from build123d import *

# Parameters (mm, degrees)
SKETCH1_W               = 25
SKETCH1_H               = 70
SKETCH1_R               = 7.6
SKETCH1_R_2             = 5.25
BOSS_EXTRUDE2_DEPTH     = 100
SKETCH1_12_R            = 1.575
CUT_EXTRUDE5_DEPTH      = 12.8
SKETCH1_27_R            = 11.15
CORTAR_EXTRUIR1_DEPTH   = 3.5
CROQUIS1_W              = 70
CROQUIS1_H              = 25
SALIENTE_EXTRUIR1_DEPTH = 150
CROQUIS4_R              = 29
CORTAR_EXTRUIR2_DEPTH   = 30
CUT_EXTRUDE6_START      = -25
CROQUIS4_3_W            = 12.3
CROQUIS4_3_H            = 22.718001441
CUT_EXTRUDE6_DEPTH      = 22
CUT_EXTRUDE7_START      = -25
CROQUIS4_4_R            = 1
CUT_EXTRUDE7_DEPTH      = 6
SKETCH2_W               = 12.2
SKETCH2_H               = 6.16
CUT_EXTRUDE11_DEPTH     = 28
CROQUIS5_R              = 2.6
CORTAR_EXTRUIR3_DEPTH   = 50


with BuildPart() as part:
    # Sketch1 → Boss-Extrude2 (new body)
    with BuildSketch(Plane(origin=(0, 0, 0), x_dir=(1, 0, 0), z_dir=(0, 1, 0))):
        Rectangle(SKETCH1_W, SKETCH1_H)
        with Locations((0, 21)):
            Circle(SKETCH1_R, mode=Mode.SUBTRACT)
        with Locations((0, -21)):
            Circle(SKETCH1_R, mode=Mode.SUBTRACT)
        Circle(SKETCH1_R_2, mode=Mode.SUBTRACT)
    extrude(amount=BOSS_EXTRUDE2_DEPTH)

    # Sketch1<12> → Cut-Extrude5 (cut)
    with BuildSketch(Plane(origin=(0, 0, 0), x_dir=(1, 0, 0), z_dir=(0, 1, 0))):
        with Locations((0, 8.193732966)):
            Circle(SKETCH1_12_R)
        with Locations((8.193732966, 0)):
            Circle(SKETCH1_12_R)
        with Locations((0, -8.193732966)):
            Circle(SKETCH1_12_R)
        with Locations((-8.193732966, 0)):
            Circle(SKETCH1_12_R)
    extrude(amount=CUT_EXTRUDE5_DEPTH, mode=Mode.SUBTRACT)

    # Sketch1<27> → Cortar-Extruir1 (cut)
    with BuildSketch(Plane(origin=(0, 0, 0), x_dir=(1, 0, 0), z_dir=(0, 1, 0))):
        Circle(SKETCH1_27_R)
    extrude(amount=CORTAR_EXTRUIR1_DEPTH, mode=Mode.SUBTRACT)

    # Croquis1 → Saliente-Extruir1 (add)
    with BuildSketch(Plane(origin=(12.5, 0, 0), x_dir=(0, 0, -1), z_dir=(1, 0, 0))):
        with Locations((0, 12.5)):
            Rectangle(CROQUIS1_W, CROQUIS1_H)
    extrude(amount=SALIENTE_EXTRUIR1_DEPTH)

    # Croquis4 → Cortar-Extruir2 (cut)
    with BuildSketch(Plane.XZ):
        with Locations((107.66, 0)):
            Circle(CROQUIS4_R)
    extrude(amount=-CORTAR_EXTRUIR2_DEPTH, mode=Mode.SUBTRACT)

    # Croquis4<3> → Cut-Extrude6 (cut)
    with BuildSketch(Plane.XZ.offset(CUT_EXTRUDE6_START)):
        with Locations((32.807294184, 12.912589049)):
            Rectangle(CROQUIS4_3_W, CROQUIS4_3_H)
    extrude(amount=CUT_EXTRUDE6_DEPTH, mode=Mode.SUBTRACT)

    # Croquis4<4> → Cut-Extrude7 (cut)
    with BuildSketch(Plane.XZ.offset(CUT_EXTRUDE7_START)):
        with Locations((32.807294184, -1.398410231)):
            Circle(CROQUIS4_4_R)
        with Locations((32.807294184, 26.301614952)):
            Circle(CROQUIS4_4_R)
    extrude(amount=CUT_EXTRUDE7_DEPTH, mode=Mode.SUBTRACT)

    # Sketch2 → Cut-Extrude11 (cut)
    with BuildSketch(Plane.XY.offset(35)):
        with Locations((32.75, 11.48)):
            Rectangle(SKETCH2_W, SKETCH2_H)
    extrude(amount=-CUT_EXTRUDE11_DEPTH, mode=Mode.SUBTRACT)

    # Croquis5 → Cortar-Extruir3 (cut)
    with BuildSketch(Plane(origin=(0, 25, 0), x_dir=(1, 0, 0), z_dir=(0, 1, 0))):
        with Locations((56.60021437, -13.16922633)):
            Circle(CROQUIS5_R)
        with Locations((56.60021437, 11.27722458)):
            Circle(CROQUIS5_R)
    extrude(amount=-CORTAR_EXTRUIR3_DEPTH, mode=Mode.SUBTRACT)


solid = part.part
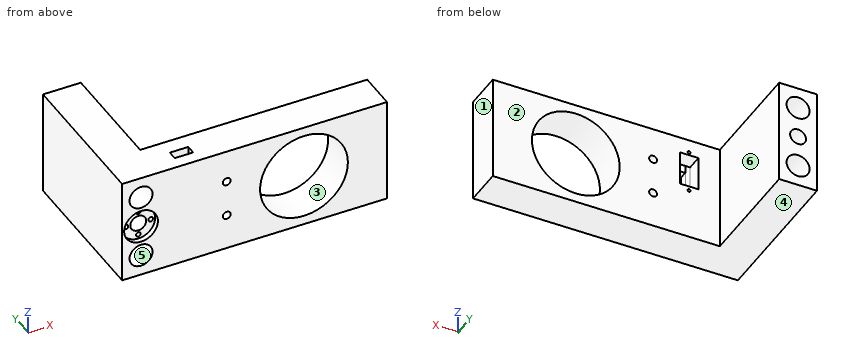
Work out the finished part from the listing and answer in its coordinate system (mm). Face numbers are marked on the shaded views. A direction names the side the tool comes from. Give positions to 0.01 mm unless a question says otherwise; leave off trailing zeros. Write each loop counter-clockwise with the first axis right and the second up, starting at its lowest first coordinate (ties: lowest second). Pieces come first, ordered by that corner, then holes. Notation, with made-up numbers: (68.5, 5) - (85.5, 5) arc R25 cw to (85.5, 31) - close; hole circle Ø7 at (10, -18). An arc over 180 degrees is marked (long way). One line per item, written item: value. Start each with the question number.
1. Find section D-D (z = 21). State how many separate pieces and enclosed holes the cut face has, then the cut area to 3 significant figures.
2. For the marked faces 1 and 2, determine the directions among +Z, -Z, +X, -X, +Y, -Y from which every point of the face is accessible in a straight line to the end or side of a thin tool.
3. For a pull along X with two mould halves and no side action, classify the marked faces 3, 4, 5 and 6 as +X half, -X half, draft (parallel to the pull), parting line (faces both ways), or undercut.
4. Find section C-C (y = 82.5). Write down the section's boundary in (x, z).
5. Find section B-B (z = -21). Write down the section's boundary in (x, y), then the cut area to 3 significant figures.
6. Given pin 1 (13.5 mm diameter, centred on x = 33.5, z = 22, fed in from +Y); pin 2 (6 mm diameter, centred on y = 48.5, z = -7, fed in from +X); pin 3 (3 mm diameter, centred on x = 56.6, z = -11.28, fed in from -Y); pin 4 (1 mm diameter, centred on x = 33, z = 26, fed in from +Y), each flat-ended and moving along its own axis, determine where each tip first touches the part or whether it passes through.
7. Find section A-A (x = 107.66). Write down the section's boundary in (y, z), then the cut area to 3 significant figures.
8. Consider probe 1 along Z at (x, y) = (0, 2.3); probe 2 along Z at (x, y) = (0, 38.5); probe 3 along X at (y, z) = (24.5, -10.5). Determine where each line is inside the solid, lowest interval first.
Geometry results:
1. separate pieces: 3
1. enclosed holes: 0
1. area: 3,460 mm2
2. face 1: +Z, -Z, +X, +Y, -Y
2. face 2: +Z, -Z, +X, +Y
3. face 3: undercut
3. face 4: draft
3. face 5: undercut
3. face 6: +X half
4. outline: (-12.5, -35) - (12.5, -35) - (12.5, 35) - (-12.5, 35) - close; hole circle Ø15.2 at (0, -21); hole circle Ø15.2 at (0, 21); hole circle Ø10.5 at (0, 0)
5. outline: (-12.5, 0) - (-7.6, 0) - (-7.6, 100) - (-12.5, 100) - close; (7.6, 0) - (87.66, 0) - (87.66, 25) - (12.5, 25) - (12.5, 100) - (7.6, 100) - close; (127.66, 0) - (162.5, 0) - (162.5, 25) - (127.66, 25) - close
5. area: 3,730 mm2
6. pin 1: y = 25
6. pin 2: x = 12.5
6. pin 3: through
6. pin 4: y = 19
7. outline: (0, -35) - (25, -35) - (25, -29) - (0, -29) - close; (0, 29) - (25, 29) - (25, 35) - (0, 35) - close
7. area: 300 mm2
8. probe 1: -35 to -28.6, -13.4 to -11.15, 11.15 to 13.4, 28.6 to 35
8. probe 2: -35 to -28.6, -13.4 to -5.25, 5.25 to 13.4, 28.6 to 35
8. probe 3: -12.5 to 54.12, 59.08 to 80.63, 134.69 to 162.5
